Can you work these out from the model? Positions are in its coordinate system, mm. Give positions to 0.01 mm unless a question says otherwise; leave off trailing zeros. Loops run counter-clockwise (first coordinate to the right, second up) from the corner with the lowest first, then second, coordinate; pieces in that order, holes last. Notation, with made-up numbers: (26, -34.5) - (54, -34.5) arc R12 cw to (54, -18.5) - close; hole circle Ø4 at (21.5, -23). An arc over 180 degrees is marked (long way). Answer as a JSON object with one key per item and string values.
```python
from build123d import *

# Parameters (mm, degrees)
SKETCH_1_R      = 2.5
EXTRUDE_1_DEPTH = 95
FILLET_1_R      = 10


with BuildPart() as part:
    # 草图1 → 凸台-拉伸1 (new body)
    with BuildSketch(Plane.XY):
        with BuildLine():
            Line((0, 50), (0, 80))
            ThreePointArc((0, 80), (30.614674589, 73.910362601), (56.568542495, 56.568542495))
            Line((56.568542495, 56.568542495), (35.355339059, 35.355339059))
            ThreePointArc((35.355339059, 35.355339059), (19.134171618, 46.193976626), (0, 50))
        make_face()
        with Locations((23.70806473, 60.410770511)):
            Circle(SKETCH_1_R, mode=Mode.SUBTRACT)
    extrude(amount=EXTRUDE_1_DEPTH)

    # 圆角1
    fillet_1_edges = [part.edges().sort_by_distance(p)[0] for p in [
        (56.568542495, 56.568542495, 47.5),
        (35.355339059, 35.355339059, 47.5),
        (0, 50, 47.5),
        (0, 80, 47.5),
    ]]
    fillet(fillet_1_edges, radius=FILLET_1_R)


solid = part.part
```
1) Imagine slicing it at C-C on x = 36.5. Write out the boundary of the cut face in (y, z).
Check sheet entries:
{"outline": "(39.06, 0) - (71.19, 0) - (71.19, 95) - (39.06, 95) - close"}
2) Imagine slicing it at D-D on y = 55. Write out the boundary of the cut face in (x, z), and give its area (3 significant figures).
Check sheet entries:
{"outline": "(0.91, 0) - (51.86, 0) - (51.86, 95) - (0.91, 95) - close", "area": "4,840 mm2"}
3) I'm going to push flat-ended pins straight in: P1, Ø4.5, axis at x = 23.71, y = 60.41, coming from the -Z side; P2, Ø12, axis at x = 42.5, z = 40, coming from the -Y side; P3, Ø5, axis at y = 75, z = 78, coming from the -X side; P4, Ø4, axis at x = 44, z = 62.5, coming from the +Y side. Where does each tip first touch, or does it pass through?
Check sheet entries:
{"P1": "through", "P2": "y = 39.06", "P3": "x = 0.53", "P4": "y = 68.09"}
4) If we mould it in two halves opening along X, with no side actions, what happens to faces 1 (the cylindrical face through (21.865, 62.1, 46.835)), 2 (the cylindrical face through (2.3, 52.78, 48.16)), 3 (the cylindrical face through (51.884, 56.897, 48.165))? For each: released by +X, released by -X, zero draft, split by the parting line, or undercut.
Check sheet entries:
{"face 1": "undercut", "face 2": "released by -X", "face 3": "released by +X"}
5) Imagine slicing it at B-B on y = 61.5. Write out the boundary of the cut face in (x, z).
Check sheet entries:
{"outline": "(0, 0) - (21.46, 0) - (21.46, 95) - (0, 95) - close; (25.96, 0) - (50.31, 0) - (50.31, 95) - (25.96, 95) - close"}
6) I need wall thicknesses on L1, parallel to Y at x = 22.5, z = 83; L2, parallel to Y at x = 35.5, z = 43; L3, parallel to X at y = 71, z = 80.5. Which ranges of each line are inside material? Lowest first, please.
Check sheet entries:
{"L1": "44.65 to 58.22, 62.6 to 76.77", "L2": "38.93 to 71.69", "L3": "0.15 to 36.86"}
7) Imagine slicing it at A-A on z = 57.5. Write out the boundary of the cut face in (x, y), and give its area (3 significant figures).
Check sheet entries:
{"outline": "(0, 59.16) arc R10 ccw to (8.33, 49.3) arc R50 cw to (28.97, 40.75) arc R10 ccw to (41.83, 41.83) - (48.99, 48.99) arc R10 ccw to (47.91, 64.07) arc R80 ccw to (11.43, 79.18) arc R10 ccw to (0, 69.28) - close; hole circle Ø5 at (23.71, 60.41)", "area": "1,430 mm2"}
